Geometry: final body of the model. Coordinates: model frame, mm. Coordinates: 2 decimals unless noted, no trailing zeros. Loops run counter-clockwise (first coordinate to the right, second up) from the corner with the lowest first, then second, coordinate; pieces in that order, holes last. Notation, with made-up numbers: (38.5, 30.5) -> (60.5, 30.5) arc R19 cw to (60.5, 43.5) -> close; hole circle Ø7 at (73.5, 40). An arc over 180 degrees is marked (long way). One line per item, written item: value. Start each with the question number.
Item 1: Section query A-A on x = 2. Return loops of the section in (y, z), then the cut area to 3 significant figures.
Item 2: Section query C-C on y = -8. Return loops of the section in (x, z), then the cut area to 3 significant figures.
Item 3: Ray query, probe 1 along Y at (x, z) = (2, 2.5); probe 2 along Y at (x, z) = (15, 1); probe 3 along X at (y, z) = (7.75, 1.95). Return the intervals inside material, ascending. Write a range as from..to.
Item 4: Contact query for a flat-ended pin moving along its axis: pin 1 Ø4 at (x, y) = (-37.5, 3.5) entering from -Z. Output: stop coordinate, or through.
Item 5: Section query B-B on z = 1.1. Return loops of the section in (x, y), then the cut area to 3 significant figures.
Item 6: Section query D-D on x = 16. Return loops of the section in (y, z), then the cut area to 3 significant figures.
from build123d import *

# Parameters (mm, degrees)
BOSS_EXTRUDE1_DEPTH = 4
SKETCH2_R           = 2.6
CUT_EXTRUDE1_DEPTH  = 4
SKETCH3_R           = 1.5
CUT_EXTRUDE2_DEPTH  = 4
FILLET1_R           = 3
SKETCH4_W           = 40
SKETCH4_H           = 20
BOSS_EXTRUDE2_DEPTH = 4
SKETCH5_R           = 1.5
CUT_EXTRUDE3_DEPTH  = 4
SKETCH6_W           = 36.661625307
SKETCH6_H           = 3
CUT_EXTRUDE4_DEPTH  = 4


with BuildPart() as part:
    # Sketch1 → Boss-Extrude1 (new body)
    with BuildSketch(Plane.XY):
        with BuildLine():
            Line((-15, 10), (-15, -10))
            Line((-15, -10), (15, -10))
            ThreePointArc((15, -10), (5, 0), (15, 10))
            Line((15, 10), (-15, 10))
        make_face()
        with BuildLine():
            ThreePointArc((15, 10), (5, 0), (15, -10))
            Line((15, -10), (15, 10))
        make_face()
        with BuildLine():
            Line((15, 10), (15, -10))
            ThreePointArc((15, -10), (22.071067812, -7.071067812), (25, 0))
            ThreePointArc((25, 0), (22.071067812, 7.071067812), (15, 10))
        make_face()
    extrude(amount=BOSS_EXTRUDE1_DEPTH)

    # Sketch2 → Cut-Extrude1 (cut)
    with BuildSketch(Plane.XY.offset(4)):
        with Locations((15, 0)):
            Circle(SKETCH2_R)
    extrude(amount=-CUT_EXTRUDE1_DEPTH, mode=Mode.SUBTRACT)

    # Sketch3 → Cut-Extrude2 (cut)
    with BuildSketch(Plane.XY.offset(4)):
        with Locations((-10, 0)):
            Circle(SKETCH3_R)
        with Locations((2, 0)):
            Circle(SKETCH3_R)
    extrude(amount=-CUT_EXTRUDE2_DEPTH, mode=Mode.SUBTRACT)

    # Fillet1
    fillet1_edges = [part.edges().sort_by_distance(p)[0] for p in [
        (-15, -10, 2),
        (-15, 10, 2),
    ]]
    fillet(fillet1_edges, radius=FILLET1_R)

    # Sketch4 → Boss-Extrude2 (add)
    with BuildSketch(Plane.XY.offset(4)):
        with Locations((-32, 0)):
            Rectangle(SKETCH4_W, SKETCH4_H)
    extrude(amount=-BOSS_EXTRUDE2_DEPTH)

    # Sketch5 → Cut-Extrude3 (cut)
    with BuildSketch(Plane.XY.offset(4)):
        with Locations((-46.661625307, 0)):
            Circle(SKETCH5_R)
    extrude(amount=-CUT_EXTRUDE3_DEPTH, mode=Mode.SUBTRACT)

    # Sketch6 → Cut-Extrude4 (cut)
    with BuildSketch(Plane.XY.offset(4)):
        with Locations((-28.330812654, 0)):
            Rectangle(SKETCH6_W, SKETCH6_H)
    extrude(amount=-CUT_EXTRUDE4_DEPTH, mode=Mode.SUBTRACT)


solid = part.part
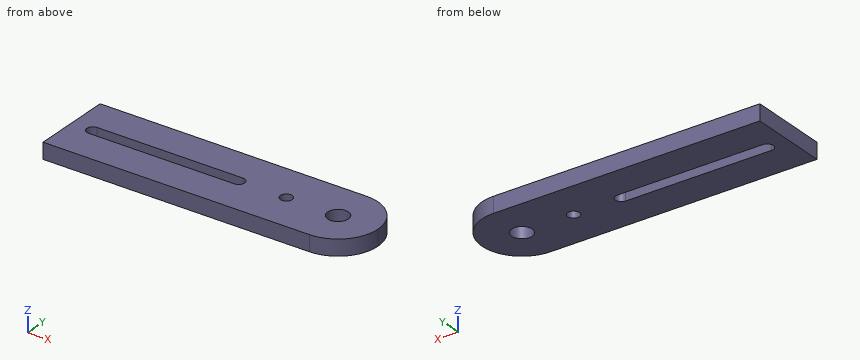
Reply:
1. outline: (-10, 0) -> (-1.5, 0) -> (-1.5, 4) -> (-10, 4) -> close; (1.5, 0) -> (10, 0) -> (10, 4) -> (1.5, 4) -> close
1. area: 68.0 mm²
2. outline: (-52, 0) -> (21, 0) -> (21, 4) -> (-52, 4) -> close
2. area: 292 mm²
3. probe 1: y = -10..-1.5, 1.5..10
3. probe 2: y = -10..-2.6, 2.6..10
3. probe 3: x = -52..21.32
4. pin 1: stops at z = 0
5. outline: (-52, -10) -> (15, -10) arc R10 ccw to (15, 10) -> (-52, 10) -> close; hole (-46.66, -1.5) -> (-10, -1.5) arc R1.5 ccw to (-10, 1.5) -> (-46.66, 1.5) arc R1.5 ccw to start; hole circle Ø3 at (2, 0); hole circle Ø5.2 at (15, 0)
5. area: 1,350 mm²
6. outline: (-9.95, 0) -> (-2.4, 0) -> (-2.4, 4) -> (-9.95, 4) -> close; (2.4, 0) -> (9.95, 0) -> (9.95, 4) -> (2.4, 4) -> close
6. area: 60.4 mm²
